Work out the finished part from the listing and answer in its coordinate system (mm). Round coordinates to 2 decimals unless told otherwise and drop trailing zeros. Write each loop counter-clockwise with the first axis right and the second up, starting at its lowest first coordinate (ties: lowest second). Pieces come first, ordered by that corner, then holes. Notation, with made-up numbers: (81.25, -28.5) -> (137.25, -28.5) arc R32 ccw to (137.25, 10.5) -> close; hole circle Ø2 at (84, 10.5). An arc over 180 degrees is marked (long way). One line per question, with ' | ' between items. Start each with the question number.
```python
from build123d import *

# Parameters (mm, degrees)
SKETCH1_W           = 250
SKETCH1_H           = 221.085663757
SKETCH1_R           = 2.5
SKETCH1_W_2         = 33
SKETCH1_H_2         = 90
BOSS_EXTRUDE1_DEPTH = 5
SKETCH6_R           = 62.5
CUT_EXTRUDE4_DEPTH  = 6


with BuildPart() as part:
    # Sketch1 → Boss-Extrude1 (new body)
    with BuildSketch(Plane.XY):
        with Locations((-3368.041949546, -177.462013972)):
            Rectangle(SKETCH1_W, SKETCH1_H)
        with Locations((-3489.041949546, -217.319182093)):
            Circle(SKETCH1_R, mode=Mode.SUBTRACT)
        with Locations((-3489.041949546, -166.319182093)):
            Circle(SKETCH1_R, mode=Mode.SUBTRACT)
        with Locations((-3247.041949546, -166.319182093)):
            Circle(SKETCH1_R, mode=Mode.SUBTRACT)
        with Locations((-3247.041949546, -217.319182093)):
            Circle(SKETCH1_R, mode=Mode.SUBTRACT)
        with Locations((-3445.601949546, -191.819182093)):
            Rectangle(SKETCH1_W_2, SKETCH1_H_2, mode=Mode.SUBTRACT)
        with Locations((-3290.481949546, -191.819182093)):
            Rectangle(SKETCH1_W_2, SKETCH1_H_2, mode=Mode.SUBTRACT)
    extrude(amount=BOSS_EXTRUDE1_DEPTH)

    # Sketch6 → Cut-Extrude4 (cut, through all)
    with BuildSketch(Plane.XY):
        with Locations((-3368.041949546, -300.417289182)):
            Circle(SKETCH6_R)
        Polygon((-3503.457885375, -270.451546314), (-3493.041949546, -264.270843991), (-3478.958452604, -288.00484585), (-3489.374388434, -294.185548172), align=None)
        with BuildLine():
            Line((-3493.041949546, -161.319182093), (-3493.041949546, -66.919182093))
            Line((-3493.041949546, -66.919182093), (-3382.503777097, -66.919182093))
            ThreePointArc((-3382.503777097, -66.919182093), (-3396.600008581, -117.423811459), (-3444.198590493, -139.419182093))
            Line((-3444.198590493, -139.419182093), (-3467.101949546, -139.419182093))
            Line((-3467.101949546, -139.419182093), (-3467.101949546, -161.319182093))
            Line((-3467.101949546, -161.319182093), (-3493.041949546, -161.319182093))
        make_face()
        Polygon((-3246.709510658, -294.185548172), (-3257.125446487, -288.00484585), (-3243.041949546, -264.270843991), (-3232.626013716, -270.451546314), align=None)
        with BuildLine():
            Line((-3268.981949546, -139.419182093), (-3291.885308598, -139.419182093))
            ThreePointArc((-3291.885308598, -139.419182093), (-3339.48389051, -117.423811459), (-3353.580121995, -66.919182093))
            Line((-3353.580121995, -66.919182093), (-3243.041949546, -66.919182093))
            Line((-3243.041949546, -66.919182093), (-3243.041949546, -161.319182093))
            Line((-3243.041949546, -161.319182093), (-3268.981949546, -161.319182093))
            Line((-3268.981949546, -161.319182093), (-3268.981949546, -139.419182093))
        make_face()
    extrude(amount=CUT_EXTRUDE4_DEPTH, mode=Mode.SUBTRACT)


solid = part.part
```
(1) A cutting plane is placed at A-A, the plane y = -203.5. Determine the outline of the cut face in (x, z).
(2) The mould has two halves that part along X. Classify faces 1 (the flat face through (-3370, -200, 5)), 2 (the cylindrical face through (-3366.84, -237.93, 2.46)), 3 (the flat face through (-3486.1, -275.97, 2.46)): +X half, -X half, draft (parallel to the pull), parting line (faces both ways), or undercut.
(3) Given pin 1 Ø2.5 at (x, z) = (-3442.5, 2) entering from +Y; pin 2 Ø1.5 at (y, z) = (-151.5, 3.5) entering from +X; pin 3 Ø1.5 at (x, z) = (-3282, 3.5) entering from +Y; pin 4 Ø3 at (x, y) = (-3464, -160.5) entering from -Z, each flat-ended and moving along its own axis, determine where each tip first touches the part or whether it passes through.
(4) A cutting plane is placed at C-C, the plane z = 3.4. Determine the outline of the cut face in (x, y), then the cut area to 3 significant figures.
(5) A cutting plane is placed at B-B, the plane x = -3433. Determine the outline of the cut face in (y, z).
(6) A cutting plane is placed at D-D, the plane y = -242.5. Determine the outline of the cut face in (x, z).
(7) Consider L1, parallel to X at y = -224, z = 1.55; L2, parallel to X at y = -155.5, z = 2.05; L3, parallel to Y at x = -3459, z = 0.8. Determine where each line is inside the solid, lowest interval first.
Returned:
1) outline: (-3493.04, 0) -> (-3462.1, 0) -> (-3462.1, 5) -> (-3493.04, 5) -> close; (-3429.1, 0) -> (-3306.98, 0) -> (-3306.98, 5) -> (-3429.1, 5) -> close; (-3273.98, 0) -> (-3243.04, 0) -> (-3243.04, 5) -> (-3273.98, 5) -> close
2) face 1: draft | face 2: undercut | face 3: -X half
3) pin 1: y = -139.35 | pin 2: x = -3268.98 | pin 3: y = -139.42 | pin 4: z = 0
4) outline: (-3493.04, -264.27) -> (-3478.96, -288) -> (-3429.3, -288) arc R62.5 cw to (-3306.79, -288) -> (-3257.13, -288) -> (-3243.04, -264.27) -> (-3243.04, -161.32) -> (-3268.98, -161.32) -> (-3268.98, -139.42) -> (-3291.89, -139.42) arc R62.5 cw to (-3353.58, -66.92) -> (-3382.5, -66.92) arc R62.5 cw to (-3444.2, -139.42) -> (-3467.1, -139.42) -> (-3467.1, -161.32) -> (-3493.04, -161.32) -> close; hole circle Ø5 at (-3489.04, -217.32); hole circle Ø5 at (-3489.04, -166.32); hole (-3462.1, -236.82) -> (-3429.1, -236.82) -> (-3429.1, -146.82) -> (-3462.1, -146.82) -> close; hole (-3306.98, -236.82) -> (-3273.98, -236.82) -> (-3273.98, -146.82) -> (-3306.98, -146.82) -> close; hole circle Ø5 at (-3247.04, -217.32); hole circle Ø5 at (-3247.04, -166.32) | area: 28,700 mm2
5) outline: (-288, 0) -> (-236.82, 0) -> (-236.82, 5) -> (-288, 5) -> close; (-146.82, 0) -> (-138.41, 0) -> (-138.41, 5) -> (-146.82, 5) -> close
6) outline: (-3493.04, 0) -> (-3391.53, 0) -> (-3391.53, 5) -> (-3493.04, 5) -> close; (-3344.55, 0) -> (-3243.04, 0) -> (-3243.04, 5) -> (-3344.55, 5) -> close
7) L1: -3493.04 to -3462.1, -3429.1 to -3306.98, -3273.98 to -3243.04 | L2: -3467.1 to -3462.1, -3429.1 to -3306.98, -3273.98 to -3268.98 | L3: -288 to -236.82, -146.82 to -139.42
